```python
from build123d import *

# Parameters (mm, degrees)
CROQUIS1_W              = 70
CROQUIS1_H              = 70
SALIENTE_EXTRUIR1_DEPTH = 20
CROQUIS2_W              = 40
CROQUIS2_H              = 40
CORTAR_EXTRUIR1_DEPTH   = 2
CROQUIS3_W              = 4
CROQUIS3_H              = 4
CORTAR_EXTRUIR2_DEPTH   = 55


with BuildPart() as part:
    # Croquis1 → Saliente-Extruir1 (new body)
    with BuildSketch(Plane(origin=(0, 0, 0), x_dir=(1, 0, 0), z_dir=(0, 1, 0))):
        with Locations((35, 35)):
            Rectangle(CROQUIS1_W, CROQUIS1_H)
    extrude(amount=SALIENTE_EXTRUIR1_DEPTH)

    # Croquis2 → Cortar-Extruir1 (cut)
    with BuildSketch(Plane(origin=(0, 20, 0), x_dir=(1, 0, 0), z_dir=(0, 1, 0))):
        with Locations((35, 35)):
            Rectangle(CROQUIS2_W, CROQUIS2_H)
    extrude(amount=-CORTAR_EXTRUIR1_DEPTH, mode=Mode.SUBTRACT)

    # Croquis3 → Cortar-Extruir2 (cut)
    with BuildSketch(Plane(origin=(0, 18, 0), x_dir=(1, 0, 0), z_dir=(0, 1, 0))):
        with Locations((47.5, 22.5)):
            Rectangle(CROQUIS3_W, CROQUIS3_H)
    extrude(amount=-CORTAR_EXTRUIR2_DEPTH, mode=Mode.SUBTRACT)


solid = part.part
```
The listing builds one solid part. Answer for the finished solid, in the listing's coordinates (mm). A direction names the side the tool comes from. Give positions to 0.01 mm unless a question says otherwise; leave off trailing zeros. Order: outer loops, then holes, each group sorted by start corner. A loop starts at its lowest first (then second) coordinate and runs counter-clockwise, first axis right, second up.
Item 1: The part is cut by section A-A, the plane z = -22. Give the vertices of the cut face in (x, y), and give its area (3 significant figures).
From the geometry:
outline: (0, 0) - (45.5, 0) - (45.5, 18) - (15, 18) - (15, 20) - (0, 20) - close; (49.5, 0) - (70, 0) - (70, 20) - (55, 20) - (55, 18) - (49.5, 18) - close
area: 1,250 mm2
Item 2: Find the intervals of material crossed by probe 1 along X at (y, z) = (6.25, -23); probe 2 along Y at (x, z) = (24, -44), in increasing order.
From the geometry:
probe 1: x = 0 to 45.5, 49.5 to 70
probe 2: y = 0 to 18
Item 3: The part is cut by section B-B, the plane x = 31. Give the vertices of the cut face in (y, z), and give its area (3 significant figures).
From the geometry:
outline: (0, -70) - (20, -70) - (20, -55) - (18, -55) - (18, -15) - (20, -15) - (20, 0) - (0, 0) - close
area: 1,320 mm2
Item 4: For a pull along Z with two mould halves and no side action, classify faces 1 (the face through (35, 19, -15)), 2 (the face through (35, 10, 0)), 3 (the face through (11, 20, -35)), 4 (the face through (55, 19, -35)) as pulls with the +Z half, pulls with the -Z half, needs draft (parallel to the pull), parting line crosses it, or undercut.
From the geometry:
face 1: undercut
face 2: pulls with the +Z half
face 3: needs draft
face 4: undercut
Item 5: The part is cut by section C-C, the plane z = -32.5. Give the vertices of the cut face in (x, y).
From the geometry:
outline: (0, 0) - (70, 0) - (70, 20) - (55, 20) - (55, 18) - (15, 18) - (15, 20) - (0, 20) - close
Item 6: Given pin 1 Ø4 at (x, z) = (26.5, -48.5) entering from +Y, flat-ended and moving along its own axis, determine where the tip first touches the part or whether it passes through.
From the geometry:
pin 1: stops at y = 18
Item 7: Which of the six approach directions +Z, -Z, +X, -X, +Y, -Y give full straight-line access (tool end or side, diameter ignored) to faces 5 (the face through (0, 10, -35)), 6 (the face through (49.5, 9, -22)), 7 (the face through (15, 19, -35))?
From the geometry:
face 5: +Z, -Z, -X, +Y, -Y
face 6: +Y, -Y
face 7: +Y
